from build123d import *

# Parameters (mm, degrees)
EXTRUDE_2_DEPTH          = 1.5
FILLET_1_R               = 1
SKETCH_3_R               = 1.6
CUT_EXTRUDE_1_DEPTH      = 223.320913296
CUT_EXTRUDE_2_DEPTH      = 223.320913296
CUT_EXTRUDE_2_DEPTH_BACK = 223.320913296
SKETCH_4_R               = 1.6
SKETCH_5_R               = 1
CUT_EXTRUDE_3_DEPTH      = 223.320913296
PATTERN_CIRCULAR_1_COUNT = 3


with BuildPart() as part:
    # Sketch 1 → Extrude 2 (new, symmetric)
    with BuildSketch(Plane(origin=(0, 0, 0), x_dir=(1, 0, 0), z_dir=(0, 1, 0))):
        with BuildLine():
            Line((97.009839672, -102.774028853), (137.509839672, -32.625971147))
            Line((137.509839672, -32.625971147), (144.908849563, 31.451334131))
            ThreePointArc((144.908849563, 31.451334131), (145.184524529, 32.21121649), (145.772298281, 32.76613982))
            Line((145.772298281, 32.76613982), (158.000220729, 39.825934137))
            Line((158.000220729, 39.825934137), (113.490381057, 116.919237886))
            Line((113.490381057, 116.919237886), (101.262458609, 109.85944357))
            ThreePointArc((101.262458609, 109.85944357), (100.487994031, 109.627878233), (99.692079121, 109.769077889))
            Line((99.692079121, 109.769077889), (40.5, 135.4))
            Line((40.5, 135.4), (-40.5, 135.4))
            Line((-40.5, 135.4), (-99.692079121, 109.769077889))
            ThreePointArc((-99.692079121, 109.769077889), (-100.487994031, 109.627878233), (-101.262458609, 109.85944357))
            Line((-101.262458609, 109.85944357), (-113.490381057, 116.919237886))
            Line((-113.490381057, 116.919237886), (-158.000220729, 39.825934137))
            Line((-158.000220729, 39.825934137), (-145.772298281, 32.76613982))
            ThreePointArc((-145.772298281, 32.76613982), (-145.184524529, 32.21121649), (-144.908849563, 31.451334131))
            Line((-144.908849563, 31.451334131), (-137.509839672, -32.625971147))
            Line((-137.509839672, -32.625971147), (-97.009839672, -102.774028853))
            Line((-97.009839672, -102.774028853), (-45.216770441, -141.22041202))
            ThreePointArc((-45.216770441, -141.22041202), (-44.696530497, -141.839094723), (-44.509839672, -142.62558339))
            Line((-44.509839672, -142.62558339), (-44.509839672, -156.745172024))
            Line((-44.509839672, -156.745172024), (44.509839672, -156.745172024))
            Line((44.509839672, -156.745172024), (44.509839672, -142.62558339))
            ThreePointArc((44.509839672, -142.62558339), (44.696530497, -141.839094723), (45.216770441, -141.22041202))
            Line((45.216770441, -141.22041202), (97.009839672, -102.774028853))
        make_face()
    extrude(amount=EXTRUDE_2_DEPTH, both=True)

    # Fillet 1
    fillet_1_edges = [part.edges().sort_by_distance(p)[0] for p in [
        (-158.000220729, 0, -39.825934137),
        (-113.490381057, 0, -116.919237886),
        (-40.5, 0, -135.4),
        (40.5, 0, -135.4),
        (113.490381057, 0, -116.919237886),
        (158.000220729, 0, -39.825934137),
        (137.509839672, 0, 32.625971147),
        (97.009839672, 0, 102.774028853),
        (44.509839672, 0, 156.745172024),
        (-44.509839672, 0, 156.745172024),
        (-97.009839672, 0, 102.774028853),
        (-137.509839672, 0, 32.625971147),
    ]]
    fillet(fillet_1_edges, radius=FILLET_1_R)

    # Sketch 3 → Cut-Extrude 1 (cut, symmetric)
    with BuildSketch(Plane.XZ.offset(1.5)):
        with Locations(Location((111.750110365, -104.933475144, 0), (0, 0, 270))):
            Circle(SKETCH_3_R)
        with Locations(Location((146.750110365, -44.311696879, 0), (0, 0, 90))):
            Circle(SKETCH_3_R)
    cut_extrude_1 = extrude(amount=CUT_EXTRUDE_1_DEPTH, both=True, mode=Mode.SUBTRACT)

    # Mirror 1: Cut-Extrude 1 across plane
    add(cut_extrude_1.mirror(Plane(origin=(0, 0, 0), x_dir=(0, 0, 1), z_dir=(1, 0, 0))), mode=Mode.SUBTRACT)

    # Sketch 4 → Cut-Extrude 2 (cut, two sides: drawn at the far end of the back side and taken through both)
    with BuildSketch(Plane.XZ.offset(1.5).offset(-CUT_EXTRUDE_2_DEPTH_BACK)):
        with Locations(Location((37.500160328, 149.245172024, 0), (0, 0, 270))):
            Circle(SKETCH_4_R)
        with Locations(Location((-37.499839672, 149.250171422, 0), (0, 0, 270))):
            Circle(SKETCH_4_R)
    extrude(amount=CUT_EXTRUDE_2_DEPTH + CUT_EXTRUDE_2_DEPTH_BACK, mode=Mode.SUBTRACT)

    # Sketch 5 → Cut-Extrude 3 (cut, symmetric)
    with BuildSketch(Plane(origin=(0, 1.5, 0), x_dir=(1, 0, 0), z_dir=(0, 1, 0))):
        with Locations(Location((-98.329077559, -40.489041807, 0), (0, 0, 270))):
            Circle(SKETCH_5_R)
        with Locations(Location((-115.649585635, -50.489041807, 0), (0, 0, 270))):
            Circle(SKETCH_5_R)
        with Locations(Location((-101.549585635, -74.910958193, 0), (0, 0, 270))):
            Circle(SKETCH_5_R)
        with Locations(Location((-84.229077559, -64.910958193, 0), (0, 0, 270))):
            Circle(SKETCH_5_R)
        Polygon((-115.621124665, -45.738337651), (-102.457538528, -38.138337651), (-98.357538528, -45.239745962), (-111.521124665, -52.839745962), align=None)
        Polygon((-101.521124665, -70.160254038), (-97.421124665, -77.261662349), (-84.257538528, -69.661662349), (-88.357538528, -62.560254038), align=None)
    cut_extrude_3 = extrude(amount=CUT_EXTRUDE_3_DEPTH, both=True, mode=Mode.SUBTRACT)

    # Pattern Circular 1: Cut-Extrude 3 ×3 about axis
    pattern_circular_1_axis = Axis((0, 0, 0), (0, 1, 0))
    for i in range(1, PATTERN_CIRCULAR_1_COUNT):
        add(cut_extrude_3.rotate(pattern_circular_1_axis, i * 360 / PATTERN_CIRCULAR_1_COUNT), mode=Mode.SUBTRACT)


solid = part.part
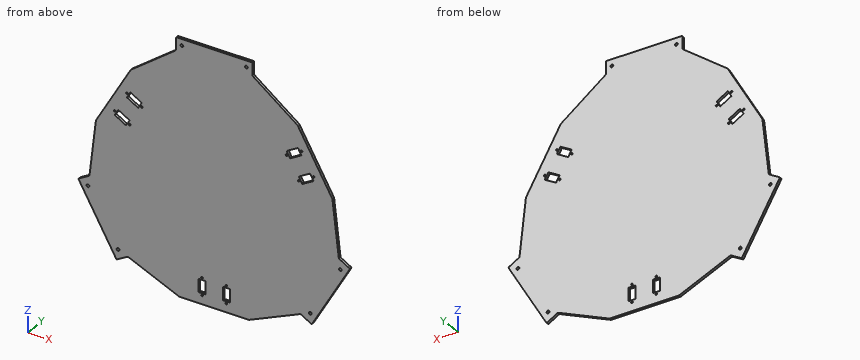
Work out the finished part from the listing and answer in its coordinate system (mm). Give positions to 0.01 mm unless a question says otherwise; leave off trailing zeros. Write each loop counter-clockwise with the first axis right and the second up, starting at its lowest first coordinate (ties: lowest second). Pieces come first, ordered by that corner, then holes.
Q1. The part is cut by section B-B on z = 114. Give the vertices of the cut face in (x, y), and give its area (3 significant figures).
Answer:
outline: (-81.89, -1.5) - (81.89, -1.5) - (81.89, 1.5) - (-81.89, 1.5) - close
area: 491 mm2
Q2. The part is cut by section D-D on x = 64. Give the vertices of the cut face in (y, z), and give its area (3 significant figures).
Answer:
outline: (-1.5, -125.22) - (1.5, -125.22) - (1.5, 127.28) - (-1.5, 127.28) - close
area: 758 mm2
Q3. The part is cut by section C-C on y = 0.45. State how many separate pieces and enclosed holes the cut face has, and give its area (3 significant figures).
Answer:
separate pieces: 1
enclosed holes: 24
area: 66,100 mm2
Q4. Straight lines are drawn through the part: L1, parallel to Z at x = 14.1, y = -0.4; L2, parallel to X at y = -0.3, z = -125.4; L3, parallel to Z at x = -11.5, y = 0.4. For each, find the intervals that lie inside material, in ascending order.
Answer:
L1: z = -135.4 to -126.4, -124.4 to -123, -107.8 to -106.4, -104.4 to 156.75
L2: x = -63.59 to -15.1, -13.1 to 13.1, 15.1 to 63.59
L3: z = -135.4 to -123, -107.8 to 156.75
Q5. The part is cut by section A-A on x = -92.5. Give the vertices of the cut face in (y, z), and give its area (3 significant figures).
Answer:
outline: (-1.5, -112.88) - (1.5, -112.88) - (1.5, 64.95) - (-1.5, 64.95) - close; (-1.5, 74.42) - (1.5, 74.42) - (1.5, 106.12) - (-1.5, 106.12) - close
area: 629 mm2
Q6. Given pin 1 (1.5 mm diameter, centred on y = -0.5, z = -62, fed in from -X); pin 2 (1.2 mm diameter, centred on x = -101.55, z = 74.91, fed in from -Y); pin 3 (1 mm diameter, centred on x = 117.5, y = 0, fed in from +Z); pin 4 (1.5 mm diameter, centred on y = 0, z = 147, fed in from -X), each flat-ended and moving along its own axis, determine where each tip first touches the part or whether it passes through.
Answer:
pin 1: stops at x = -145.63
pin 2: passes through
pin 3: stops at z = 68.15
pin 4: stops at x = -44.51
